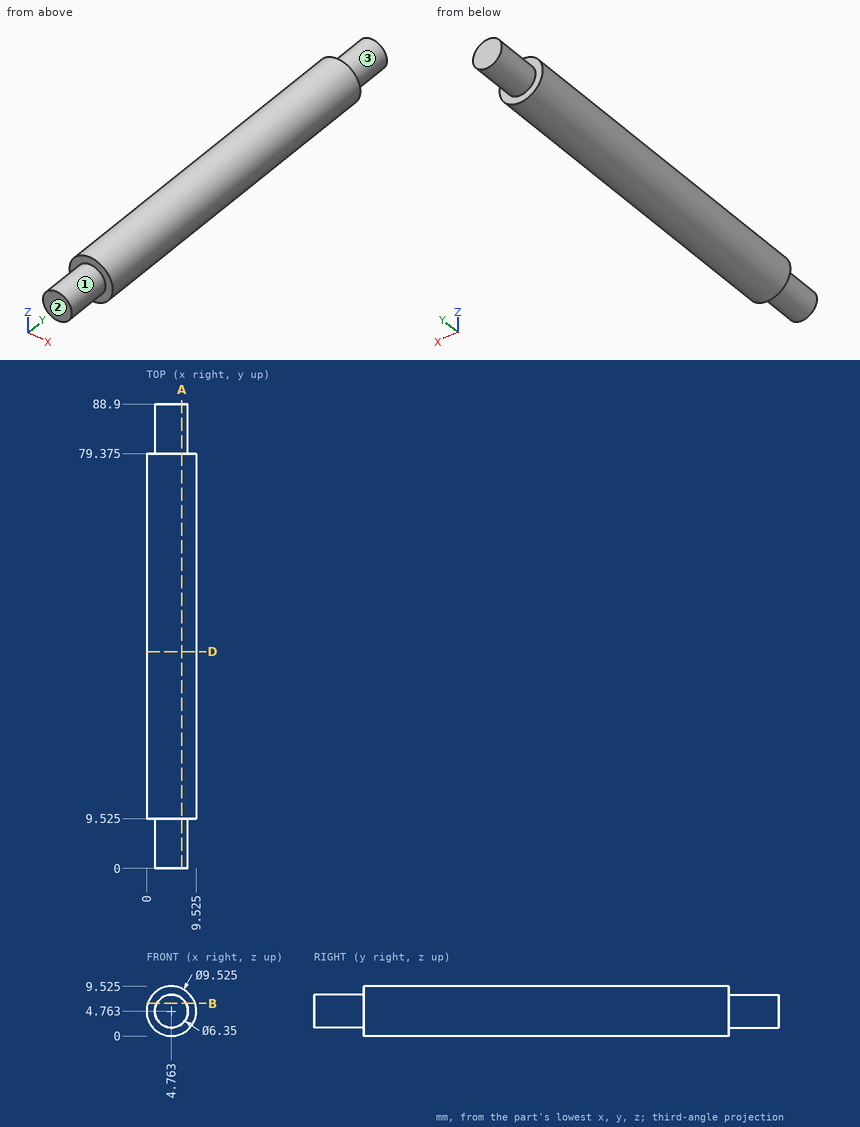
Can you work these out from the drawing? Everything is in mm from the part's minimum corner. A direction names the side the tool comes from. Coordinates: 2 decimals unless noted, no trailing zeros. Loops run counter-clockwise (first coordinate to the right, second up) from the corner with the lowest first, then second, coordinate; pieces in that order, holes last. Notation, with made-up numbers: (23.5, 70.25) - (38.5, 70.25) arc R34 ccw to (38.5, 108.25) - close; hole circle Ø2 at (33.5, 32). An arc over 180 degrees is marked (long way). Use a Markdown table: item, result.
Item 1: I want a section at A-A on x = 6.75. Please give me the cut outline in (y, z) (1 decimal).
Numbers:
| item | result |
|---|---|
| outline | (0, 2.3) - (9.5, 2.3) - (9.5, 0.4) - (79.4, 0.4) - (79.4, 2.3) - (88.9, 2.3) - (88.9, 7.2) - (79.4, 7.2) - (79.4, 9.1) - (9.5, 9.1) - (9.5, 7.2) - (0, 7.2) - close |
Item 2: Will these pins go through, and if not, where does the flat tip stop? pin 1 (2 mm diameter, centred on x = 3, y = 53.5, fed in from +Z); pin 2 (2 mm diameter, centred on x = 3, y = 43.5, fed in from -Z); pin 3 (2 mm diameter, centred on y = 10.5, z = 1, fed in from -X).
Numbers:
| item | result |
|---|---|
| pin 1 | stops at z = 9.46 |
| pin 2 | stops at z = 0.06 |
| pin 3 | stops at x = 0.88 |
Item 3: If I drill on probe 1 along Z at (x, y) = (4.75, 85.5); probe 2 along Z at (x, y) = (4.5, 26.5); probe 3 along Y at (x, z) = (3, 8.75) (1 decimal), over which ranges is the centre line in solid material (lowest first)? Write a range as from..to.
Numbers:
| item | result |
|---|---|
| probe 1 | z = 1.59..7.94 |
| probe 2 | z = 0.01..9.52 |
| probe 3 | y = 9.5..79.4 |
Item 4: For the marked faces 1, 2 and 3, which set-ups out of +Z, -Z, +X, -X, +Y, -Y let a thin tool reach every point of the face, with its end or its side?
Numbers:
| item | result |
|---|---|
| face 1 | -Y |
| face 2 | +Z, -Z, +X, -X, -Y |
| face 3 | +Y |
Item 5: I want a section at D-D on y = 41.5. Please give me the cut outline in (x, z) (1 decimal).
Numbers:
| item | result |
|---|---|
| outline | circle Ø9.5 at (4.8, 4.8) |
Item 6: I want a section at B-B on z = 6.25. Please give me the cut outline in (x, y) (1 decimal), and give its area (3 significant figures).
Numbers:
| item | result |
|---|---|
| outline | (0.2, 9.5) - (2, 9.5) - (2, 0) - (7.6, 0) - (7.6, 9.5) - (9.3, 9.5) - (9.3, 79.4) - (7.6, 79.4) - (7.6, 88.9) - (2, 88.9) - (2, 79.4) - (0.2, 79.4) - close |
| area | 739 mm2 |
